Work out the finished part from the listing and answer in its coordinate system (mm). A direction names the side the tool comes from. Coordinates: 2 decimals unless noted, no trailing zeros. Order: outer loops, then holes, each group sorted by start corner. A loop starts at its lowest first (then second) coordinate and runs counter-clockwise, first axis right, second up. Notation, with made-up numbers: M -32.5,86.5 L 7.5,86.5 A16 ccw 7.5,93.5 Z; hole C 17,58.5 d5. An arc over 180 degrees is marked long. Use a Markdown table: item, result. Add a question column.
Autodesk Inventor part; units mm, degrees
ref_plane "YZ Plane" through (0, 0, 0) normal (1, 0, 0) x (0, 1, 0)
ref_plane "XZ Plane" through (0, 0, 0) normal (0, 1, 0) x (-1, 0, 0)
ref_plane "XY Plane" through (0, 0, 0) normal (0, 0, 1) x (1, 0, 0)
ref_plane "作業平面1" through (0, 0, 0) normal (0, 0, 1) x (1, 0, 0)
sketch "スケッチ1" plane through (0, 0, 0) normal (0, 0, 1) x (1, 0, 0)
  arc A0 (9.4, -12.7373) -> (9.4, 12.7373) centre (12, 0) ccw
  circle A1 centre (10.8888, 11) radius 0.8
  circle A2 centre (10.8888, -11) radius 0.8
  circle A3 centre (10.8888, 11) radius 2
  circle A4 centre (10.8888, -11) radius 2
  arc A5 (12.8328, -11.4698) -> (12.8328, 11.4698) centre (12, 0) ccw
  line L0 (9.4, 12.7373) -> (-19.4, 6.8586)
  line L1 (-19.4, -6.8586) -> (9.4, -12.7373)
  line L2 (-1.4086, 10.5311) -> (-1.1086, 9.0614)
  line L3 (-1.1086, 9.0614) -> (8.8914, 11.1026)
  line L4 (-1.4086, -10.5311) -> (-1.1086, -9.0614)
  line L5 (-1.1086, -9.0614) -> (8.8914, -11.1026)
  point P0 (0, 0)
  point P1 (10.1875, -12.873)
  point P2 (11.2013, -12.9754)
  point P3 (11.2013, 12.9754)
  point P4 (10.1875, 12.873)
  dimension "d0" = 4
  dimension "d1" = 1.5
  dimension "d2" = 1.5
  dimension "d3" = 10
extrude "押し出し1" add sketch "スケッチ1" along normal blind 5
properties part number "MotorCover"
(1) A cutting plane is placed at A-A on x = 12. Write down the section's boundary in (y, z).
(2) A cutting plane is placed at D-D on x = 1. Write down the section's boundary in (y, z).
(3) Which of the six approach directions +Z, -Z, +X, -X, +Y, -Y give full straight-line access (tool end or side, diameter ignored) to faces 4 (the flat face through (3.821, -10.068, 2.465)), 5 (the cylindrical face through (10.68, 12.99, 2.46)), 6 (the flat face through (-1.26, 9.81, 2.46))?
(4) Straight lines are drawn through the part: line 1 (Y direction, x = 10.75, z = 3.55); line 2 (Y direction, x = 18.5, z = 1.9); line 3 (Y direction, x = 10, z = 1.25). For each, find the intervals that lie inside material, in ascending order.
(5) A cutting plane is placed at C-C on y = 0. Write down the section's boundary in (x, z), plus the area to 3 significant figures.
(6) Given P1, Ø1, axis at x = 12.5, z = 3, coming from the +Y side; P2, Ø1, axis at x = 19, z = 3.5, coming from the -Y side, each flat-ended and moving along its own axis, determine where each tip first touches the part or whether it passes through.
(7) The mould has two halves that part along X. Classify faces 1 (the flat face through (3.92, -11.62, 2.46)), 2 (the flat face through (3.821, 10.068, 2.465)), 3 (the flat face through (12, -10, 0)): pulls with the +X half, pulls with the -X half, needs draft (parallel to the pull), parting line crosses it, or undercut.
From the geometry:
| question | item | result |
|---|---|---|
| 1 | outline | M -13,0 L -9.34,0 L -9.34,5 L -13,5 Z; M 9.34,0 L 13,0 L 13,5 L 9.34,5 Z |
| 2 | outline | M -11.02,0 L -9.49,0 L -9.49,5 L -11.02,5 Z; M 9.49,0 L 11.02,0 L 11.02,5 L 9.49,5 Z |
| 3 | face 4 | +Z, -Z |
| 3 | face 5 | +Z, -Z, +Y |
| 3 | face 6 | +Z, -Z, -X |
| 4 | line 1 | y = -13 to -11.79, -10.21 to -9, 9 to 10.21, 11.79 to 13 |
| 4 | line 2 | y = -11.26 to -9.49, 9.49 to 11.26 |
| 4 | line 3 | y = -12.85 to -9.21, 9.21 to 12.85 |
| 5 | outline | M 23.5,0 L 25,0 L 25,5 L 23.5,5 Z |
| 5 | area | 7.50 mm2 |
| 6 | P1 | stops at y = 13 |
| 6 | P2 | stops at y = -11.26 |
| 7 | face 1 | pulls with the -X half |
| 7 | face 2 | undercut |
| 7 | face 3 | needs draft |
